Geometry check sheet. Reference: the model listing, model coordinates, mm. Round coordinates to 2 decimals unless told otherwise and drop trailing zeros. Loops run counter-clockwise (first coordinate to the right, second up) from the corner with the lowest first, then second, coordinate; pieces in that order, holes last. Notation, with made-up numbers: (77, 3.5) - (102, 3.5) arc R21 ccw to (102, 19.5) - close; hole circle Ø8 at (73, 64). An arc over 180 degrees is marked (long way). Answer as CSV lines item,"result". Start each with the question number.
1) Thickness scan on line 1 along Y through (x, z) = (0, 0.65); line 2 along X through (y, z) = (-2, 0.2); line 3 along Y through (x, z) = (6.5, 1.45). Record the ranges inside material, lowest first.
2) Cross-section at A-A on x = 0. Record the boundary of the cut face in (y, z), and give its area (3 significant figures).
3) Cross-section at C-C on z = 1. Record the boundary of the cut face in (x, y), and give its area (3 significant figures).
4) Cross-section at B-B on y = -25. Record the boundary of the cut face in (x, z).
5) Cross-section at D-D on x = -33.5. Record the boundary of the cut face in (y, z), and give its area (3 significant figures).
6) Draft check along X on faces 1 (the cylindrical face through (-4.067, 30.976, 1.252)), 2 (the flat face through (-9.071, -46, 1)), 3 (the flat face through (-3, -47.979, 1)), 4 (the flat face through (3.629, -46, 1)). Enter one of: released by +X, released by -X, zero draft, split by the parting line, or undercut.
7) Depth check by flat-ended pin: P1, Ø1, axis at y = -11.5, z = 0.5, coming from the -X side; P2, Ø0.8, axis at y = -46, z = 1, coming from the -X side; P3, Ø1.3, axis at y = -47, z = 2, coming from the +X side. Enter the tip coordinate at first touch or a pass-through.
from build123d import *

# Parameters (mm, degrees)
F0_R     = 31.242
F1_DEPTH = 2.54


with BuildPart() as f1:
    # F0 (on Top) → F1 (new body)
    with BuildSketch(Plane.XY):
        with BuildLine():
            ThreePointArc((3.628571, -44.301647), (32.688626, -30.120695), (44.45, 0))
            ThreePointArc((44.45, 0), (-28.040841, 34.489328), (-9.071429, -43.5145))
            ThreePointArc((-9.071429, -43.5145), (-2.749741, -44.364867), (3.628571, -44.301647))
        make_face()
        Circle(F0_R, mode=Mode.SUBTRACT)
        with BuildLine():
            ThreePointArc((3.628571, -44.301647), (-2.749741, -44.364867), (-9.071429, -43.5145))
            Line((-9.071429, -43.5145), (-9.071429, -47.97935))
            Line((-9.071429, -47.97935), (3.628571, -47.97935))
            Line((3.628571, -47.97935), (3.628571, -44.301647))
        make_face()
    extrude(amount=F1_DEPTH)


solid = f1.part
Answer block:
1,line 1,"y = -47.98 to -31.24, 31.24 to 44.45"
1,line 2,"x = -44.4 to -31.18, 31.18 to 44.4"
1,line 3,"y = -43.97 to -30.56, 30.56 to 43.97"
2,outline,"(-47.98, 0) - (-31.24, 0) - (-31.24, 2.54) - (-47.98, 2.54) - close; (31.24, 0) - (44.45, 0) - (44.45, 2.54) - (31.24, 2.54) - close"
2,area,"76.1 mm^2"
3,outline,"(-9.07, -47.98) - (3.63, -47.98) - (3.63, -44.3) arc R44.45 ccw to (44.45, 0) arc R44.45 ccw (long way) to (-9.07, -43.51) - close; hole circle Ø62.48 at (0, 0)"
3,area,"3,190 mm^2"
4,outline,"(-36.75, 0) - (-18.74, 0) - (-18.74, 2.54) - (-36.75, 2.54) - close; (18.74, 0) - (36.75, 0) - (36.75, 2.54) - (18.74, 2.54) - close"
5,outline,"(-29.22, 0) - (29.22, 0) - (29.22, 2.54) - (-29.22, 2.54) - close"
5,area,"148 mm^2"
6,face 1,"undercut"
6,face 2,"released by -X"
6,face 3,"zero draft"
6,face 4,"released by +X"
7,P1,"stops at x = -43.07"
7,P2,"stops at x = -9.07"
7,P3,"stops at x = 3.63"
